CAD build for the part. Positions are in the model's coordinates, mm. A direction names the side the tool comes from. Give positions to 0.01 mm unless a question says otherwise; leave off trailing zeros. Write each loop counter-clockwise with the first axis right and the second up, starting at its lowest first coordinate (ties: lowest second). Pieces come first, ordered by that corner, then holes. Notation, with made-up numbers: (-11.75, -13.5) - (-7.75, -13.5) arc R24 cw to (-7.75, 0.5) - close; hole circle Ø1 at (-33, 36). An arc over 180 degrees is marked (long way). Put each result on its own line as item: value. Start each with the question number.
1. Drop flat-ended pins along their axis: pin 1 (8 mm diameter, centred on x = 9, y = 39, fed in from +Z); pin 2 (10 mm diameter, centred on x = 26.5, z = 7.5, fed in from +Y); pin 3 (10 mm diameter, centred on x = 8.5, z = 18, fed in from -Y). Give the stop position or say it passes through.
2. Cut at A-A on z = 20. List the corners of the cut face in (x, y).
3. Cut at D-D on z = -15.5. List the corners of the cut face in (x, y).
4. Mould opens along Y. For faces 4 (the cylindrical face through (0.57, 12.4, 15.8)), 5 (the flat face through (15, 45, -25.5)), 6 (the flat face through (15, 0, -10)), 7 (the cylindrical face through (2.2, 56.4, -12.5)) say: +Y half, -Y half, draft (parallel to the pull), parting line (faces both ways), or undercut.
5. Cut at C-C on x = 9. List the corners of the cut face in (y, z), and give its area (3 significant figures).
6. Cut at B-B on y = 56.5. List the corners of the cut face in (x, z).
7. Tool access for faces 1 (the cylindrical face through (0.57, 84.4, -15.18)), 2 (the flat face through (15, 4, 10)), 3 (the flat face through (14.8, 84, -3.5)): list every direction of +Z, -Z, +X, -X, +Y, -Y with a clear straight run to the whole face (end or side of a thin tool).
8. Wall check: line 1 (Z direction, x = 15, y = 8.7); line 2 (Y direction, x = 1.75, z = -15); line 3 (Z direction, x = 6.25, y = 42). Give the ranges that are in metal, low to high.
Autodesk Inventor part; units mm, degrees
ref_plane "YZ Plane" through (0, 0, 0) normal (1, 0, 0) x (0, 1, 0)
ref_plane "XZ Plane" through (0, 0, 0) normal (0, 1, 0) x (-1, 0, 0)
ref_plane "XY Plane" through (0, 0, 0) normal (0, 0, 1) x (1, 0, 0)
sketch "Sketch1" plane through (0, 0, 0) normal (1, 0, 0) x (0, 1, 0)
  line L0 (0, 0) -> (0, -30)
  line L1 (13, 0) -> (30, 0) construction
  line L2 (0, -30) -> (85, -30)
  line L3 (13, 0) -> (85, 0)
  line L4 (85, 0) -> (85, -30)
  line L5 (0, 0) -> (0, 10)
  line L6 (13, 0) -> (14, 0) construction
  line L7 (0, 10) -> (8, 10)
  line L8 (8, 10) -> (8, 30)
  line L9 (8, 30) -> (13, 30)
  line L10 (13, 30) -> (13, 0)
  point P0 (59, -15)
  dimension "d0" = 30
  dimension "d2" = 85
  dimension "d4" = 10
  dimension "d6" = 8
  dimension "d7" = 20
  dimension "d8" = 5
  dimension "d47" = 30
extrude "Extrusion1" add sketch "Sketch1" along normal blind 30
sketch "Sketch2" plane through (0, 85, 0) normal (0, 1, 0) x (1, 0, 0)
  line L0 (4.5, 4.5) -> (4.5, 25.5)
  line L1 (4.5, 4.5) -> (25.5, 4.5) construction
  line L2 (4.5, 25.5) -> (25.5, 25.5)
  line L3 (25.5, 25.5) -> (25.5, 4.5)
  line L4 (25.5, 4.5) -> (4.5, 4.5)
  line L5 (30, 30) -> (30, 0)
  point P0 (0, 0)
  dimension "d13" = 21
  dimension "d14" = 90
  dimension "d15" = 21
  dimension "d16" = 90
  dimension "d17" = 21
  dimension "d18" = 90
  dimension "d19" = 21
  dimension "d46" = 4.5
  dimension "d48" = 90
  dimension "d49" = 4.5
extrude "Extrusion2" cut sketch "Sketch2" against normal blind 80
fillet "Fillet1" radius 2 12 edges at (30, 85, -15) (15, 85, 0) (15, 85, -30) (0, 85, -15) (30, 49, 0) (30, 42.5, -30) (0, 49, 0) (0, 42.5, -30) (0, 13, 15) (15, 13, 30) (30, 13, 15) (15, 13, 0)
sketch "Sketch4" plane through (2, 13, 2) normal (0, 1, 0) x (1, 0, 0)
  line L0 (-2, -28) -> (28, -28)
  point P0 (-2, 2)
  point P1 (13, -18)
  point P2 (13, -28)
  dimension "d37" = 10
hole "Hole1" at (15, 13, 20) direction (0, -1, 0) diameter 5 end through all countersink diameter 10 countersink angle 77.33
sketch "Sketch6" plane through (30, 0, 0) normal (1, 0, 0) x (0, 0, -1)
  line L0 (-10, 0) -> (28, 0)
  point P0 (0, 0)
  point P1 (15, 56.5)
  dimension "d45" = 56.5
hole "Hole2" at (30, 56.5, -15) direction (-1, 0, 0) diameter 5 end through all
chamfer "Chamfer2" distance 2 angle 45 4 edges at (4.5, 85, -15) (15, 85, -25.5) (25.5, 85, -15) (15, 85, -4.5)
fillet "Fillet3" radius 2 4 edges at (3.5, 84, -26.5) (26.5, 84, -26.5) (26.5, 84, -3.5) (3.5, 84, -3.5)
properties part number "flexibler_standfuß_v0.8"
Report:
1. pin 1: stops at z = 0
1. pin 2: stops at y = 13
1. pin 3: stops at y = 8
2. outline: (0, 8) - (12.5, 8) - (12.5, 9.88) - (10, 13) - (2, 13) arc R2 ccw to (0, 11) - close; (17.5, 8) - (30, 8) - (30, 11) arc R2 ccw to (28, 13) - (20, 13) - (17.5, 9.88) - close
3. outline: (0, 0) - (30, 0) - (30, 54.05) - (25.5, 54.05) - (25.5, 5) - (4.5, 5) - (4.5, 54.05) - (0, 54.05) - close; (0, 58.95) - (4.5, 58.95) - (4.5, 83) - (2.5, 85) - (2, 85) arc R2 ccw to (0, 83) - close; (25.5, 58.95) - (30, 58.95) - (30, 83) arc R2 ccw to (28, 85) - (27.5, 85) - (25.5, 83) - close
4. face 4: +Y half
4. face 5: draft
4. face 6: -Y half
4. face 7: undercut
5. outline: (0, -30) - (83, -30) arc R2 ccw to (85, -28) - (85, -27.5) - (83, -25.5) - (5, -25.5) - (5, -4.5) - (83, -4.5) - (85, -2.5) - (85, -2) arc R2 ccw to (83, 0) - (15, 0) arc R2 cw to (13, 2) - (13, 28) arc R2 ccw to (11, 30) - (8, 30) - (8, 10) - (0, 10) - close
5. area: 1,090 mm²
6. outline: (0, -28) arc R2 ccw to (2, -30) - (28, -30) arc R2 ccw to (30, -28) - (30, -17.5) - (25.5, -17.5) - (25.5, -25.5) - (4.5, -25.5) - (4.5, -17.5) - (0, -17.5) - close; (0, -12.5) - (4.5, -12.5) - (4.5, -4.5) - (25.5, -4.5) - (25.5, -12.5) - (30, -12.5) - (30, -2) arc R2 ccw to (28, 0) - (2, 0) arc R2 ccw to (0, -2) - close
7. face 1: +Z, -Z, -X, +Y
7. face 2: +Z, +X, -X, -Y
7. face 3: +Y
8. line 1: z = -30 to -25.5, -4.5 to 17.5, 22.5 to 30
8. line 2: y = 0 to 54, 59 to 84.98
8. line 3: z = -30 to -25.5, -4.5 to 0
